```python
from build123d import *

# Parameters (mm, degrees)
BOSS_EXTRUDE1_DEPTH = 1.6
BOSS_EXTRUDE2_DEPTH = 14


with BuildPart() as part:
    # Sketch1 → Boss-Extrude1 (new body)
    with BuildSketch(Plane(origin=(0, 0, 0), x_dir=(1, 0, 0), z_dir=(0, 1, 0))):
        Polygon((0, 0), (0, 15.5), (26, 15.5), (26, 17.5), (40, 17.5), (40, 0), align=None)
    extrude(amount=BOSS_EXTRUDE1_DEPTH)

    # Sketch2 → Boss-Extrude2 (add)
    with BuildSketch(Plane(origin=(0, 0, -16), x_dir=(-1, 0, 0), z_dir=(0, 0, -1))):
        Polygon((-40, 1.6), (-28.5, 1.6), (-28.5, 5), (-26.5, 5), (-26.5, 10), (-28.5, 10), (-28.5, 14.4), (-40, 14.4), align=None)
    extrude(amount=-BOSS_EXTRUDE2_DEPTH)


solid = part.part
```
Work out the finished part from the listing and answer in its coordinate system (mm). A direction names the side the tool comes from. Round coordinates to 2 decimals unless told otherwise and drop trailing zeros. Loops run counter-clockwise (first coordinate to the right, second up) from the corner with the lowest first, then second, coordinate; pieces in that order, holes last.
(1) The part is cut by section B-B, the plane x = 29.5. Give the vertices of the cut face in (y, z), and give its area (3 significant figures).
Computed values:
outline: (0, -17.5) - (1.6, -17.5) - (1.6, -16) - (14.4, -16) - (14.4, -2) - (1.6, -2) - (1.6, 0) - (0, 0) - close
area: 207 mm2
(2) The mould has two halves that part along Y. Classify faces 4 (the flat face through (28.5, 3, -9)), 5 (the flat face through (27, 10, -9)), 6 (the flat face through (26, 1, -16)): pulls with the +Y half, pulls with the -Y half, needs draft (parallel to the pull), parting line crosses it, or undercut.
Computed values:
face 4: undercut
face 5: pulls with the +Y half
face 6: needs draft
(3) For faces 1 (the flat face through (13, 1, -15.5)), 2 (the flat face through (28, 5, -9)), 3 (the flat face through (28.5, 12, -9)), determine the directions among +Z, -Z, +X, -X, +Y, -Y from which every point of the face is accessible in a straight line to the end or side of a thin tool.
Computed values:
face 1: -Z, -X, +Y, -Y
face 2: +Z, -Z, -X
face 3: +Z, -Z, -X, +Y
(4) The part is cut by section A-A, the plane z = -6. Give the vertices of the cut face in (x, y).
Computed values:
outline: (0, 0) - (40, 0) - (40, 14.4) - (28.5, 14.4) - (28.5, 10) - (26.5, 10) - (26.5, 5) - (28.5, 5) - (28.5, 1.6) - (0, 1.6) - close
(5) Find the intervals of material crossed by L1, parallel to Y at x = 28, z = -2.5; L2, parallel to X at y = 3.25, z = -6; L3, parallel to Z at x = 35.5, y = 7.25, in increasing order.
Computed values:
L1: y = 0 to 1.6, 5 to 10
L2: x = 28.5 to 40
L3: z = -16 to -2
(6) The part is cut by section C-C, the plane y = 11. Give the vertices of the cut face in (x, z), and give its area (3 significant figures).
Computed values:
outline: (28.5, -16) - (40, -16) - (40, -2) - (28.5, -2) - close
area: 161 mm2
(7) Each of these flat-tipped pins is pushed along its axis until it touches: P1, Ø2, axis at y = 12, z = -9.5, coming from the -X side; P2, Ø6, axis at y = 6.5, z = -15, coming from the -X side; P3, Ø2, axis at x = 22.5, z = -2.5, coming from the +Y side; P4, Ø5, axis at x = 19.5, z = -5.5, coming from the -Y side. Where does it stop, or does it pass through?
Computed values:
P1: stops at x = 28.5
P2: stops at x = 26.5
P3: stops at y = 1.6
P4: stops at y = 0
(8) The part is cut by section D-D, the plane x = 18.5. Give the vertices of the cut face in (y, z), and give its area (3 significant figures).
Computed values:
outline: (0, -15.5) - (1.6, -15.5) - (1.6, 0) - (0, 0) - close
area: 24.8 mm2
